Print and shaded views of the part. All mm, measured from the part's lowest x, y and z. Coordinates: 2 decimals unless noted, no trailing zeros. Order: outer loops, then holes, each group sorted by start corner. A loop starts at its lowest first (then second) coordinate and runs counter-clockwise, first axis right, second up. Notation, with made-up numbers: M 77,33.25 L 107,33.25 A27 cw 107,55.25 Z; hole C 21,30 d4. An arc over 180 degrees is marked long. Return JSON: item names as keys, results as strings.
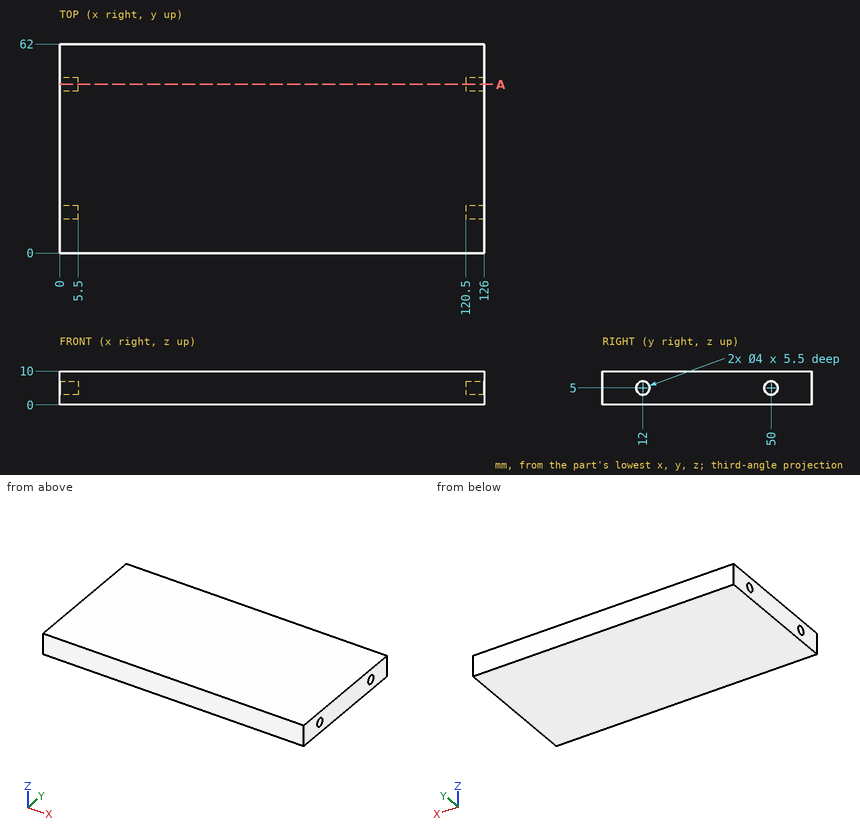
Item 1: Wall check: line 1 (Y direction, x = 1.85, z = 5); line 2 (Z direction, x = 2.45, y = 50); line 3 (X direction, y = 13.5, z = 4.5). Give the ranges that are in metal, low to high.
Check result:
{"line 1": "y = 0 to 10, 14 to 48, 52 to 62", "line 2": "z = 0 to 3, 7 to 10", "line 3": "x = 5.5 to 120.5"}
Item 2: Drop flat-ended pins along their axis: pin 1 Ø1.2 at (y, z) = (49.5, 4.5) entering from -X; pin 2 Ø3 at (y, z) = (12, 5) entering from +X. Give the stop position or say it passes through.
Check result:
{"pin 1": "stops at x = 5.5", "pin 2": "stops at x = 120.5"}
Item 3: Saw through at A-A (y = 50). Write the cut outline in (x, z), and give its area (3 significant figures).
Check result:
{"outline": "M 0,0 L 126,0 L 126,3 L 120.5,3 L 120.5,7 L 126,7 L 126,10 L 0,10 L 0,7 L 5.5,7 L 5.5,3 L 0,3 Z", "area": "1,220 mm2"}
